Autodesk Inventor part; units mm, degrees
ref_plane "YZ Plane" through (0, 0, 0) normal (1, 0, 0) x (0, 1, 0)
ref_plane "XZ Plane" through (0, 0, 0) normal (0, 1, 0) x (-1, 0, 0)
ref_plane "XY Plane" through (0, 0, 0) normal (0, 0, 1) x (1, 0, 0)
sketch "スケッチ1" plane through (0, 0, 0) normal (0, 0, 1) x (1, 0, 0)
  line L0 (0, 0) -> (43.3, 0)
  line L1 (43.3, 20) -> (0, 20)
  line L2 (0, 10) -> (43.3, 10) construction
  line L3 (43.3, 14) -> (45.3, 14)
  line L4 (45.3, 14) -> (45.3, 6)
  line L5 (45.3, 6) -> (43.3, 6)
  arc A0 (43.3, 16) -> (43.3, 14) centre (43.3, 15) ccw
  arc A1 (43.3, 6) -> (43.3, 4) centre (43.3, 5) ccw
  line L6 (43.3, 0) -> (43.3, 4)
  line L7 (43.3, 16) -> (43.3, 20)
  line L8 (21.65, 20) -> (21.65, 0) construction
  line L9 (0, 14) -> (-2, 14)
  line L10 (-2, 14) -> (-2, 6)
  line L11 (-2, 6) -> (0, 6)
  arc A2 (0, 14) -> (0, 16) centre (0, 15) ccw
  arc A3 (0, 4) -> (0, 6) centre (0, 5) ccw
  line L12 (0, 0) -> (0, 4)
  line L13 (0, 16) -> (0, 20)
  dimension "d0" = 43.3
  dimension "d1" = 20
  dimension "d5" = 8
  dimension "d6" = 2
extrude "押し出し1" add sketch "スケッチ1" along normal blind 5
sketch "スケッチ3" plane through (43.3, 0, 0) normal (1, 0, 0) x (0, 0, -1)
  line L0 (0, 0) -> (-5, 0)
  line L1 (-2.5, 0) -> (-2.5, 20) construction
  line L2 (0, 20) -> (-5, 20)
  line L3 (-2.5, 10) -> (0, 10) construction
  line L4 (0, 6) -> (0, 14)
  point P0 (-2.5, 17.5)
  point P1 (-2.5, 2.5)
  dimension "d7" = 15
hole "穴1" at (43.3, 17.5, 2.5) at (43.3, 2.5, 2.5) direction (-1, 0, 0) diameter 2.4 depth 8 tip angle 118
sketch "スケッチ4" plane through (0, 16, 0) normal (-1, 0, 0) x (0, 0, 1)
  circle A0 centre (2.5, 1.5) radius 1.2
  circle A1 centre (2.5, -13.5) radius 1.2
  circle A2 centre (2.5, -13.5) radius 1.2
  point P0 (0, -16)
hole "穴2" at (0, 17.5, 2.5) at (0, 2.5, 2.5) direction (1, 0, 0) diameter 2.4 depth 8 tip angle 118
properties part number "頭_メインフレームセンター２" material "アセタール樹脂、黒"
Input: part model. Units: mm. Frame: model coordinates. A direction names the side the tool comes from. Coordinates: 2 decimals unless noted, no trailing zeros. Write each loop counter-clockwise with the first axis right and the second up, starting at its lowest first coordinate (ties: lowest second). Pieces come first, ordered by that corner, then holes. Notation, with made-up numbers: (1.5, 88.5) -> (55.5, 88.5) arc R14 cw to (55.5, 114.5) -> close; hole circle Ø9 at (65.5, 19). An arc over 180 degrees is marked (long way). Answer as a JSON object with one key per item and string values.
1. Mould query, pull axis Z, two halves, no side actions, for faces 1 (the face through (42.3, 5, 2.5)), 2 (the face through (21, 10, 0)), 3 (the face through (4.056, 18.565, 3.054)). Classes: released by +Z, released by -Z, zero draft, split by the parting line, or undercut.
Result set:
{"face 1": "zero draft", "face 2": "released by -Z", "face 3": "undercut"}
2. Material intervals for line 1 (Y direction, x = 3.75, z = 2.5); line 2 (Z direction, x = 4.25, y = 17.5); line 3 (X direction, y = 3.5, z = 4.4), sorted ascending. Write a range as from..to.
Result set:
{"line 1": "y = 0..1.3, 3.7..16.3, 18.7..20", "line 2": "z = 0..1.3, 3.7..5", "line 3": "x = 0..43.3"}
3. Section B-B on y = 5. Return the cut outline in (x, z).
Result set:
{"outline": "(1, 0) -> (42.3, 0) -> (42.3, 5) -> (1, 5) -> close"}
4. First-contact query: P1, Ø1, axis at x = -1.5, z = 2, coming from the +Y side; P2, Ø1, axis at x = 44, z = 3, coming from the -Y side; P3, Ø1.4, axis at y = 2.5, z = 2.5, coming from the +X side. Flat tips, straight axial feed; report the tip coordinate or a pass-through.
Result set:
{"P1": "stops at y = 14", "P2": "stops at y = 6", "P3": "stops at x = 35"}
5. Access query for faces 4 (the face through (39.244, 18.565, 1.946)), 5 (the face through (44, 6, 2)), 6 (the face through (0, 1, 2)). Directions: +Z, -Z, +X, -X, +Y, -Y. A direction counts if a zero-diameter tool reaches every point of the face in a straight line with its end or side. Return the directions, or none.
Result set:
{"face 4": "+X", "face 5": "+Z, -Z, +X, -Y", "face 6": "+Z, -Z, -X, -Y"}
6. Section A-A on x = 4. Return the cut outline in (y, z), then the cut area to 3 significant figures.
Result set:
{"outline": "(0, 0) -> (20, 0) -> (20, 5) -> (0, 5) -> close; hole circle Ø2.4 at (2.5, 2.5); hole circle Ø2.4 at (17.5, 2.5)", "area": "91.0 mm2"}
